from build123d import *

# Parameters (mm, degrees)
SKETCH1_R           = 76.191937258
BOSS_EXTRUDE1_DEPTH = 75.946
BOSS_EXTRUDE2_DEPTH = 75.946


with BuildPart() as part:
    # Sketch1 → Boss-Extrude1 (new body)
    with BuildSketch(Plane.XY):
        with Locations((-25.384457056, 7.752300794)):
            Circle(SKETCH1_R)
    extrude(amount=BOSS_EXTRUDE1_DEPTH)

    # Sketch2 → Boss-Extrude2 (add)
    with BuildSketch(Plane.XY.offset(75.946)):
        Polygon((-10.949916627, 11.135298471), (-18.648882466, 24.470298471), (-34.046814146, 24.470298471), (-41.745779985, 11.135298471), (-34.046814146, -2.199701529), (-18.648882466, -2.199701529), align=None)
    extrude(amount=BOSS_EXTRUDE2_DEPTH)


solid = part.part
The listing builds one solid part. Answer for the finished solid, in the listing's coordinates (mm). A direction names the side the tool comes from. Coordinates: 2 decimals unless noted, no trailing zeros. Order: outer loops, then holes, each group sorted by start corner. A loop starts at its lowest first (then second) coordinate and runs counter-clockwise, first axis right, second up.
Q1. A cutting plane is placed at C-C, the plane x = -15.5. Write down the section's boundary in (y, z), and give its area (3 significant figures).
Q2. A cutting plane is placed at B-B, the plane y = 14. Write down the section's boundary in (x, z), and give its area (3 significant figures).
Q3. Consider line 1 (Z direction, x = -9, y = -60); line 2 (Y direction, x = -23, z = 10.5); line 3 (Y direction, x = -21, z = 129). Determine where each line is inside the solid, lowest interval first.
Q4. A cutting plane is placed at A-A, the plane z = 93.5. Write down the section's boundary in (x, y).
Q5. Given P1, Ø5, axis at x = -45.5, z = 72.5, coming from the -Y side; P2, Ø8, axis at y = 19, z = 133.5, coming from the +X side; P3, Ø2, axis at x = -19, z = 107.5, coming from the +Y side, each flat-ended and moving along its own axis, determine where each tip first touches the part or whether it passes through.
Q6. Which of the six approach directions +Z, -Z, +X, -X, +Y, -Y give full straight-line access (tool end or side, diameter ignored) to faces 1 (the face through (-26, 24.47, 113)), 2 (the face through (-37.84, 17.9, 113.39)), 3 (the face through (-37.95, 4.56, 113.39)), 4 (the face through (-14.746, 17.709, 113.387)), 5 (the face through (-14.853, 4.374, 113.387))?
Q7. A cutting plane is placed at D-D, the plane x = -75. Write down the section's boundary in (y, z), and give its area (3 significant figures).
Answers follow:
1. outline: (-67.8, 0) - (83.3, 0) - (83.3, 75.95) - (19.02, 75.95) - (19.02, 151.89) - (3.25, 151.89) - (3.25, 75.95) - (-67.8, 75.95) - close
1. area: 12,700 mm2
2. outline: (-101.32, 0) - (50.55, 0) - (50.55, 75.95) - (-12.6, 75.95) - (-12.6, 151.89) - (-40.09, 151.89) - (-40.09, 75.95) - (-101.32, 75.95) - close
2. area: 13,600 mm2
3. line 1: z = 0 to 75.95
3. line 2: y = -68.4 to 83.91
3. line 3: y = -2.2 to 24.47
4. outline: (-41.75, 11.14) - (-34.05, -2.2) - (-18.65, -2.2) - (-10.95, 11.14) - (-18.65, 24.47) - (-34.05, 24.47) - close
5. P1: stops at y = -66.38
5. P2: stops at x = -13.18
5. P3: stops at y = 24.47
6. face 1: +Z, +X, -X, +Y
6. face 2: +Z, -X, +Y
6. face 3: +Z, -X, -Y
6. face 4: +Z, +X, +Y
6. face 5: +Z, +X, -Y
7. outline: (-50.07, 0) - (65.58, 0) - (65.58, 75.95) - (-50.07, 75.95) - close
7. area: 8,780 mm2
